from build123d import *

# Parameters (mm, degrees)
BOSS_EXTRUDE1_DEPTH = 120.65
SKETCH3_R           = 14.2621
CUT_EXTRUDE1_DEPTH  = 107.95
SKETCH4_R           = 2.54
CUT_EXTRUDE2_DEPTH  = 127
SKETCH5_R           = 2.54
CUT_EXTRUDE3_DEPTH  = 127
FILLET1_R           = 2.54
FILLET2_R           = 2.54


with BuildPart() as part:
    # Sketch2 → Boss-Extrude1 (new body)
    with BuildSketch(Plane(origin=(0, 0, 0), x_dir=(1, 0, 0), z_dir=(0, 1, 0))):
        Polygon((0, 0), (41.226518858, 0), (41.226518858, -12.7), (36.248118858, -12.7), (36.248118858, -4.4704), (0, -4.4704), (-33.1216, -4.4704), (-33.1216, -12.7), (-38.1, -12.7), (-38.1, 0), align=None)
    extrude(amount=BOSS_EXTRUDE1_DEPTH)

    # Sketch3 → Cut-Extrude1 (cut)
    with BuildSketch(Plane(origin=(0, 0, 0), x_dir=(-1, 0, 0), z_dir=(0, 0, -1))):
        with Locations((-3.126518858, 101.6)):
            Circle(SKETCH3_R)
    extrude(amount=-CUT_EXTRUDE1_DEPTH, mode=Mode.SUBTRACT)

    # Sketch4 → Cut-Extrude2 (cut)
    with BuildSketch(Plane(origin=(0, 0, 0), x_dir=(-1, 0, 0), z_dir=(0, 0, -1))):
        with Locations((0, 34.925)):
            Circle(SKETCH4_R)
    extrude(amount=-CUT_EXTRUDE2_DEPTH, mode=Mode.SUBTRACT)

    # Sketch5 → Cut-Extrude3 (cut)
    with BuildSketch(Plane(origin=(0, 0, 0), x_dir=(-1, 0, 0), z_dir=(0, 0, -1))):
        with Locations((0, 6.985)):
            Circle(SKETCH5_R)
    extrude(amount=-CUT_EXTRUDE3_DEPTH, mode=Mode.SUBTRACT)

    # Fillet1
    fillet1_edges = [part.edges().sort_by_distance(p)[0] for p in [
        (-33.1216, 60.325, 4.4704),
    ]]
    fillet(fillet1_edges, radius=FILLET1_R)

    # Fillet2
    fillet2_edges = [part.edges().sort_by_distance(p)[0] for p in [
        (36.248118858, 60.325, 4.4704),
    ]]
    fillet(fillet2_edges, radius=FILLET2_R)


solid = part.part
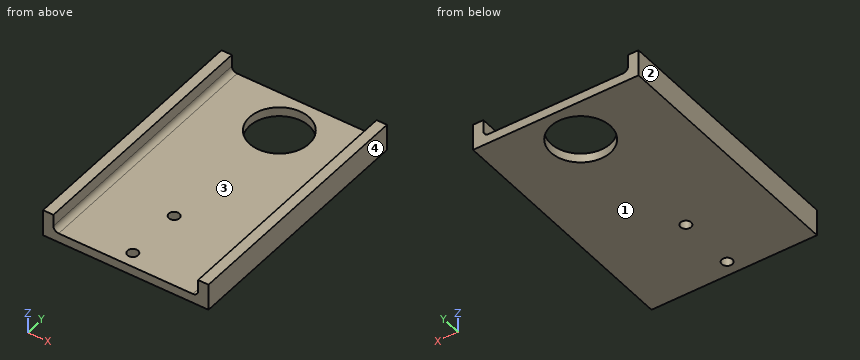
Verification items for the finished model (mm, model axes). Face numbers are marked on the shaded views. Coordinates: 2 decimals unless noted, no trailing zeros. Loops run counter-clockwise (first coordinate to the right, second up) from the corner with the lowest first, then second, coordinate; pieces in that order, holes last. Notation, with made-up numbers: (41, 37) -> (73, 37) arc R24 cw to (73, 49) -> close; hole circle Ø2 at (-2.75, 36.5). An arc over 180 degrees is marked (long way). Answer as a JSON object with one key per item and string values. Group by question number.
Item 1: Sectioned sample at A-A on y = 101.6. Record the boundary of the cut face in (x, z).
Item 2: Sectioned sample at C-C on y = 74.5. Record the boundary of the cut face in (x, z).
Item 3: Scan lines: probe 1 along X at (y, z) = (48, 10.5); probe 2 along Y at (x, z) = (0, 2.75) (3 decimals); probe 3 along Z at (x, y) = (33, 112.5). Record each from-to range of solid material in increasing order.
Item 4: Sectioned sample at D-D on x = -18. Record the boundary of the cut face in (y, z).
Item 5: Mould release check, pull along X, two halves, no side actions. Record for the marked faces 1, 2, 3 and 4: +X half, -X half, draft (parallel to the pull), parting line (faces both ways), or undercut.
Item 6: Depth check by flat-ended pin: pin 1 (6.5 mm diameter, centred on x = 0, y = 34.925, fed in from +Z); pin 2 (5 mm diameter, centred on x = -29.5, z = 10.5, fed in from +Y). Enter the tip coordinate at first touch or a pass-through.
Item 7: Sectioned sample at B-B on x = 4. Record the boundary of the cut face in (y, z).
Evaluation:
{
 "1": {"outline": "(-38.1, 0) -> (-11.14, 0) -> (-11.14, 4.47) -> (-30.58, 4.47) arc R2.54 cw to (-33.12, 7.01) -> (-33.12, 12.7) -> (-38.1, 12.7) -> close; (17.39, 0) -> (41.23, 0) -> (41.23, 12.7) -> (36.25, 12.7) -> (36.25, 7.01) arc R2.54 cw to (33.71, 4.47) -> (17.39, 4.47) -> close"},
 "2": {"outline": "(-38.1, 0) -> (41.23, 0) -> (41.23, 12.7) -> (36.25, 12.7) -> (36.25, 7.01) arc R2.54 cw to (33.71, 4.47) -> (-30.58, 4.47) arc R2.54 cw to (-33.12, 7.01) -> (-33.12, 12.7) -> (-38.1, 12.7) -> close"},
 "3": {"probe 1": "x = -38.1 to -33.12, 36.25 to 41.23", "probe 2": "y = 0 to 4.445, 9.525 to 32.385, 37.465 to 87.685, 115.515 to 120.65", "probe 3": "z = 0 to 4.47"},
 "4": {"outline": "(0, 0) -> (120.65, 0) -> (120.65, 4.47) -> (0, 4.47) -> close"},
 "5": {"face 1": "draft", "face 2": "-X half", "face 3": "undercut", "face 4": "+X half"},
 "6": {"pin 1": "stops at z = 4.47", "pin 2": "passes through"},
 "7": {"outline": "(0, 0) -> (87.36, 0) -> (87.36, 4.47) -> (0, 4.47) -> close; (115.84, 0) -> (120.65, 0) -> (120.65, 4.47) -> (115.84, 4.47) -> close"}
}
